Model file for the job. Use its own axes, mm. Coordinates: 2 decimals unless noted, no trailing zeros. Order: outer loops, then holes, each group sorted by start corner. A loop starts at its lowest first (then second) coordinate and runs counter-clockwise, first axis right, second up. Notation, with made-up numbers: (15, 72) -> (61, 72) arc R22 cw to (61, 81) -> close; hole circle Ø10 at (48, 3). An arc over 180 degrees is marked (long way). Return JSON: item names as keys, results as strings. Group by question number.
1) Cut at A-A (y = 0). Write the cut outline in (x, z), and give its area (3 significant figures).
2) Flat gauge pins, fed straight in: pin 1 (1 mm diameter, centred on x = -2, z = 28.5, fed in from -Y); pin 2 (1 mm diameter, centred on y = -1, z = 8.5, fed in from -X); pin 3 (2 mm diameter, centred on x = 2, z = 24, fed in from -Y). Where does each tip first touch, or does it go through?
3) Cut at D-D (z = 18). Write the cut outline in (x, y), and give its area (3 significant figures).
4) Cut at B-B (z = 41.5). Write the cut outline in (x, y), and give its area (3 significant figures).
5) Probe line 1 (Y direction, x = 0, z = 35.25); line 2 (X direction, y = -0.25, z = 41); line 3 (Z direction, x = -1, y = 0). List the from-to ranges inside material, lowest first.
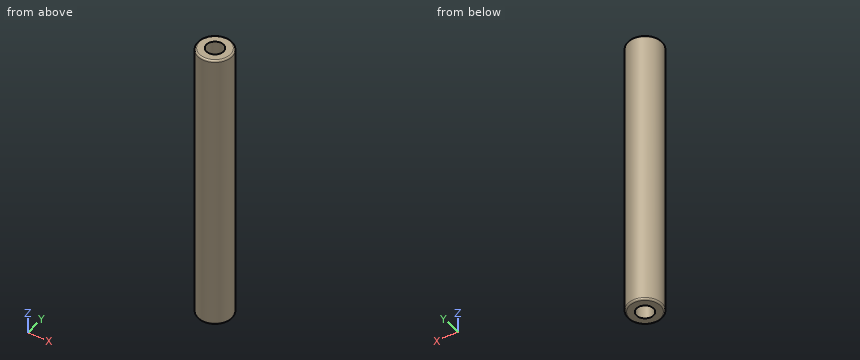
Autodesk Inventor part; units mm, degrees
ref_plane "YZ Plane" through (0, 0, 0) normal (1, 0, 0) x (0, 1, 0)
ref_plane "XZ Plane" through (0, 0, 0) normal (0, 1, 0) x (-1, 0, 0)
ref_plane "XY Plane" through (0, 0, 0) normal (0, 0, 1) x (1, 0, 0)
sketch "スケッチ1" plane through (0, 0, 0) normal (0, 0, 1) x (1, 0, 0)
  circle A0 centre (0, 0) radius 3
  circle A1 centre (0, 0) radius 1.5
  dimension "d0" = 6
  dimension "d1" = 3
extrude "押し出し1" add sketch "スケッチ1" along normal blind 50
fillet "フィレット1" radius 0.3 2 edges at (-3, 0, 50) (-3, 0, 0)
thread "ねじ1"
extrude "押し出し2" add sketch "スケッチ1" along normal blind 24 contours A1
extrude "押し出し3" cut sketch "スケッチ1" along normal blind 6 contours A1
thread "ねじ2"
properties part number "スペーサーM3L50アルミ" material "アルミニウム 2014-T4"
Answers below:
{
 "1": {"outline": "(-3, 0.3) arc R0.3 ccw to (-2.7, 0) -> (-1.5, 0) -> (-1.5, 6) -> (1.5, 6) -> (1.5, 0) -> (2.7, 0) arc R0.3 ccw to (3, 0.3) -> (3, 49.7) arc R0.3 ccw to (2.7, 50) -> (1.5, 50) -> (1.5, 24) -> (-1.5, 24) -> (-1.5, 50) -> (-2.7, 50) arc R0.3 ccw to (-3, 49.7) -> close", "area": "204 mm^2"},
 "2": {"pin 1": "stops at y = -2.6", "pin 2": "stops at x = -2.96", "pin 3": "stops at y = -2.83"},
 "3": {"outline": "circle Ø6 at (0, 0)", "area": "28.3 mm^2"},
 "4": {"outline": "circle Ø6 at (0, 0); hole circle Ø3 at (0, 0)", "area": "21.2 mm^2"},
 "5": {"line 1": "y = -3 to -1.5, 1.5 to 3", "line 2": "x = -2.99 to -1.48, 1.48 to 2.99", "line 3": "z = 6 to 24"}
}
